```python
from build123d import *

# Parameters (mm, degrees)
F1_DEPTH = 76.2
F3_DEPTH = 92.076
F4_DEPTH = 92.076
F5_W     = 6.35
F5_H     = 19.05
F6_DEPTH = 73.026
F7_W     = 6.35
F7_H     = 19.05
F8_DEPTH = 73.026


with BuildPart() as f1:
    # F0 (on Front) → F1 (new body)
    with BuildSketch(Plane.XZ):
        Polygon((0, -50.8), (0, 0), (19.05, 38.1), (69.85, 38.1), (69.85, 41.275), (17.087742, 41.275), (-3.175, 0.749516), (-3.175, -50.8), align=None)
    extrude(amount=F1_DEPTH)

    # F2 (on face) → F3 (cut, through all)
    with BuildSketch(Plane.XY.offset(41.275)):
        with BuildLine():
            ThreePointArc((53.975, -19.05), (56.220064, -18.120064), (57.15, -15.875))
            ThreePointArc((57.15, -15.875), (56.220064, -13.629936), (53.975, -12.7))
            ThreePointArc((53.975, -12.7), (50.8, -15.875), (53.975, -19.05))
        make_face()
        with BuildLine():
            ThreePointArc((53.975, -19.05), (50.8, -15.875), (53.975, -12.7))
            Line((53.975, -12.7), (34.925, -12.7))
            ThreePointArc((34.925, -12.7), (37.170064, -13.629936), (38.1, -15.875))
            ThreePointArc((38.1, -15.875), (37.170064, -18.120064), (34.925, -19.05))
            Line((34.925, -19.05), (53.975, -19.05))
        make_face()
        with BuildLine():
            ThreePointArc((38.1, -15.875), (37.170064, -13.629936), (34.925, -12.7))
            ThreePointArc((34.925, -12.7), (31.75, -15.875), (34.925, -19.05))
            ThreePointArc((34.925, -19.05), (37.170064, -18.120064), (38.1, -15.875))
        make_face()
    extrude(amount=-F3_DEPTH, mode=Mode.SUBTRACT)

    # F2 (on face) → F4 (cut, through all)
    with BuildSketch(Plane.XY.offset(41.275)):
        with BuildLine():
            ThreePointArc((38.1, -60.325), (37.170064, -58.079936), (34.925, -57.15))
            ThreePointArc((34.925, -57.15), (31.75, -60.325), (34.925, -63.5))
            ThreePointArc((34.925, -63.5), (37.170064, -62.570064), (38.1, -60.325))
        make_face()
        with BuildLine():
            ThreePointArc((53.975, -63.5), (56.220064, -62.570064), (57.15, -60.325))
            ThreePointArc((57.15, -60.325), (56.220064, -58.079936), (53.975, -57.15))
            ThreePointArc((53.975, -57.15), (50.8, -60.325), (53.975, -63.5))
        make_face()
        with BuildLine():
            ThreePointArc((53.975, -63.5), (50.8, -60.325), (53.975, -57.15))
            Line((53.975, -57.15), (34.925, -57.15))
            ThreePointArc((34.925, -57.15), (37.170064, -58.079936), (38.1, -60.325))
            ThreePointArc((38.1, -60.325), (37.170064, -62.570064), (34.925, -63.5))
            Line((34.925, -63.5), (53.975, -63.5))
        make_face()
    extrude(amount=-F4_DEPTH, mode=Mode.SUBTRACT)

    # F5 (on face) → F6 (cut, through all)
    with BuildSketch(Plane(origin=(-3.175, 0, 0), x_dir=(0, -1, 0), z_dir=(-1, 0, 0))):
        with BuildLine():
            Line((19.05, -34.925), (12.7, -34.925))
            ThreePointArc((12.7, -34.925), (15.875, -38.1), (19.05, -34.925))
        make_face()
        with BuildLine():
            ThreePointArc((19.05, -15.875), (15.875, -12.7), (12.7, -15.875))
            Line((12.7, -15.875), (19.05, -15.875))
        make_face()
        with Locations((15.875, -25.4)):
            Rectangle(F5_W, F5_H)
    extrude(amount=-F6_DEPTH, mode=Mode.SUBTRACT)

    # F7 (on face) → F8 (cut, through all)
    with BuildSketch(Plane(origin=(-3.175, 0, 0), x_dir=(0, -1, 0), z_dir=(-1, 0, 0))):
        with BuildLine():
            Line((57.15, -15.875), (63.5, -15.875))
            ThreePointArc((63.5, -15.875), (60.325, -12.7), (57.15, -15.875))
        make_face()
        with BuildLine():
            ThreePointArc((57.15, -34.925), (60.325, -38.1), (63.5, -34.925))
            Line((63.5, -34.925), (57.15, -34.925))
        make_face()
        with Locations((60.325, -25.4)):
            Rectangle(F7_W, F7_H)
    extrude(amount=-F8_DEPTH, mode=Mode.SUBTRACT)


solid = f1.part
```
Can you work these out from the model? Positions are in its coordinate system, mm. A direction names the side the tool comes from. Coordinates: 2 decimals unless noted, no trailing zeros. Loops run counter-clockwise (first coordinate to the right, second up) from the corner with the lowest first, then second, coordinate; pieces in that order, holes last.
Item 1: Suppose I cut it at B-B (z = -32). Please give me the cut outline in (x, y) (3 decimals).
Answers below:
outline: (-3.175, -76.2) - (0, -76.2) - (0, -63.5) - (-3.175, -63.5) - close; (-3.175, -57.15) - (0, -57.15) - (0, -19.05) - (-3.175, -19.05) - close; (-3.175, -12.7) - (0, -12.7) - (0, 0) - (-3.175, 0) - close
Item 2: Suppose I cut it at D-D (x = 30). Please give me the cut outline in (y, z) (3 decimals).
Answers below:
outline: (-76.2, 38.1) - (0, 38.1) - (0, 41.275) - (-76.2, 41.275) - close
Item 3: Which directions (+Z, -Z, +X, -X, +Y, -Y) give clear straight access to the entire face, cutting with the end or side of a thin tool? Please do faces 4 (the face through (-1.6, -15.9, -12.7)), 5 (the face through (45, -57.15, 40)), 6 (the face through (44, -38, 38.1)), 7 (the face through (-3.175, -38, -25)), 8 (the face through (-2, -38, -50.8)).
Answers below:
face 4: +X, -X
face 5: +Z, -Z
face 6: -Z, +X, +Y, -Y
face 7: +Z, -Z, -X, +Y, -Y
face 8: -Z, +X, -X, +Y, -Y
Item 4: Please list where these lines run through material, in increasing order: L1, parallel to X at y = -37, z = -33 (3 decimals); L2, parallel to Z at x = 30, y = -65.5 (3 decimals); L3, parallel to Z at x = 16, y = -8.
Answers below:
L1: x = -3.175 to 0
L2: z = 38.1 to 41.275
L3: z = 32 to 39.1
Item 5: If we mould it in two halves opening along X, with no side actions, what happens to faces 1 (the face through (0, -38, -26)), 2 (the face through (45, -12.7, 40)), 3 (the face through (-2, -63.5, -26))? For each: released by +X, released by -X, zero draft, split by the parting line, or undercut.
Answers below:
face 1: released by +X
face 2: undercut
face 3: zero draft
Item 6: I'm going to push flat-ended pins straight in: pin 1 (5 mm diameter, centred on y = -50.5, z = 6, fed in from -X); pin 2 (2 mm diameter, centred on y = -39.5, z = 14.5, fed in from -X); pin 3 (2 mm diameter, centred on y = -18, z = 6.5, fed in from -X). Where does each tip first touch, or does it pass through?
Answers below:
pin 1: stops at x = -1.8
pin 2: stops at x = 3.2
pin 3: stops at x = -0.8
Item 7: Suppose I cut it at A-A (x = 48.5). Please give me the cut outline in (y, z) (3 decimals).
Answers below:
outline: (-76.2, 38.1) - (-63.5, 38.1) - (-63.5, 41.275) - (-76.2, 41.275) - close; (-57.15, 38.1) - (-19.05, 38.1) - (-19.05, 41.275) - (-57.15, 41.275) - close; (-12.7, 38.1) - (0, 38.1) - (0, 41.275) - (-12.7, 41.275) - close
Item 8: Suppose I cut it at C-C (y = -31.5). Please give me the cut outline in (x, z) (3 decimals).
Answers below:
outline: (-3.175, -50.8) - (0, -50.8) - (0, 0) - (19.05, 38.1) - (69.85, 38.1) - (69.85, 41.275) - (17.088, 41.275) - (-3.175, 0.75) - close
